The model under review builds one solid part; all positions refer to its coordinate system, in mm. A direction names the side the tool comes from. Coordinates: 2 decimals unless noted, no trailing zeros. Order: outer loops, then holes, each group sorted by start corner. A loop starts at its lowest first (then second) coordinate and runs counter-clockwise, first axis right, second up. Notation, with made-up numbers: (9.5, 78.5) -> (50.5, 78.5) arc R25 ccw to (50.5, 96.5) -> close; hole circle Ø8 at (24, -19.75). An arc over 180 degrees is marked (long way). Use one line per item in the form item = value.
Autodesk Inventor part; units mm, degrees
ref_plane "YZ Plane" through (0, 0, 0) normal (1, 0, 0) x (0, 1, 0)
ref_plane "XZ Plane" through (0, 0, 0) normal (0, 1, 0) x (-1, 0, 0)
ref_plane "XY Plane" through (0, 0, 0) normal (0, 0, 1) x (1, 0, 0)
sketch "Sketch1" plane through (0, 0, 0) normal (0, 1, 0) x (-1, 0, 0)
  line L0 (0, 0) -> (-177.8, 0)
  line L1 (-177.8, 0) -> (-177.8, 254)
  line L2 (-177.8, 254) -> (0, 254)
  line L3 (0, 254) -> (0, 0)
  dimension "d0" = 177.8
  dimension "d1" = 254
extrude "Extrusion1" add sketch "Sketch1" along normal blind 57.15
shell "Shell1" thickness 3.81 removed faces 1 at (118.5333, 57.15, 169.3333)
sketch "Sketch2" plane through (0, 0, 254) normal (0, 0, 1) x (1, 0, 0)
  line L0 (0, 0) -> (177.8, 0)
  line L1 (177.8, 0) -> (177.8, 57.15)
  line L2 (0, 57.15) -> (177.8, 57.15)
  line L3 (0, 0) -> (0, 57.15)
extrude "Extrusion2" cut sketch "Sketch2" against normal up to surface (3.81 mm away)
sketch "Sketch3" plane through (3.81, 3.81, 3.81) normal (0, 1, 0) x (1, 0, 0)
  line L0 (0, -246.38) -> (170.18, -246.38)
  line L1 (170.18, -246.38) -> (170.18, 0)
  line L2 (0, 0) -> (0, -246.38)
  line L3 (170.18, -246.38) -> (-1.2603, -246.38)
  line L4 (-1.2603, -246.38) -> (-1.2603, -208.28)
  line L5 (-1.2603, -208.28) -> (170.18, -208.28)
  line L6 (170.18, -208.28) -> (170.18, -246.38)
  point P0 (-3.81, 3.81)
  point P1 (0, -208.28)
  dimension "d7" = 38.1
extrude "Extrusion3" cut sketch "Sketch3" against normal through all contours L2 L5 L1 L0
properties part number "Component box top"
Item 1: To check wall thickness, follow L1, parallel to X at y = 55.5, z = 174.5; L2, parallel to Z at x = 63, y = 16. State the ranges of each line that lie inside material, in increasing order. Write a range as from..to.
Results found:
L1 = 0..3.81, 173.99..177.8
L2 = 0..3.81
Item 2: We need section C-C (x = 132.5). Write out the cut boundary in (y, z), plus the area to 3 significant figures.
Results found:
outline = (0, 0) -> (57.15, 0) -> (57.15, 3.81) -> (3.81, 3.81) -> (3.81, 212.09) -> (0, 212.09) -> close
area = 1,010 mm²
Item 3: We need section B-B (y = 37.5). Write out the cut boundary in (x, z).
Results found:
outline = (0, 0) -> (177.8, 0) -> (177.8, 250.19) -> (173.99, 250.19) -> (173.99, 3.81) -> (3.81, 3.81) -> (3.81, 250.19) -> (0, 250.19) -> close
Item 4: Clearance check with flat-ended pins moving along their axes: pin 1 (1.5 mm diameter, centred on x = 27.5, y = 48.5, fed in from +Z); pin 2 (10 mm diameter, centred on x = 152, y = 27.5, fed in from -Z); pin 3 (1.5 mm diameter, centred on x = 18.5, z = 76.5, fed in from +Y); pin 4 (1.9 mm diameter, centred on x = 112.5, y = 2, fed in from +Z). State where each tip first meets the part, or that it passes through.
Results found:
pin_1 = 3.81
pin_2 = 0
pin_3 = 3.81
pin_4 = 212.09
Item 5: Draft analysis for pull direction X (two halves, no side actions). For faces 1 (the face through (3.81, 29, 125)), 2 (the face through (88, 28, 0)), 3 (the face through (90, 3.81, 109)), 4 (the face through (177.8, 28, 123)), state which applies: released by +X, released by -X, zero draft, split by the parting line, or undercut.
Results found:
face_1 = undercut
face_2 = zero draft
face_3 = undercut
face_4 = released by +X
Item 6: We need section A-A (z = 189.5). Write out the cut boundary in (x, y), plus the area to 3 significant figures.
Results found:
outline = (0, 0) -> (177.8, 0) -> (177.8, 57.15) -> (173.99, 57.15) -> (173.99, 3.81) -> (3.81, 3.81) -> (3.81, 57.15) -> (0, 57.15) -> close
area = 1,080 mm²
Item 7: Tool access review of faces 5 (the face through (90, 0, 127)), 6 (the face through (88, 30, 3.81)): name each direction out of +Z, -Z, +X, -X, +Y, -Y from which nothing blocks a thin tool from reaching the whole face with its end or side.
Results found:
face_5 = +Z, -Z, +X, -X, -Y
face_6 = +Z, +Y
